from build123d import *

# Parameters (mm, degrees)
F2_R    = 10.6144552681
F3_SIZE = 5


# Not quite as in the source:
# - a feature of the source that left no trace in its solid (it failed there, or was rolled back) is left out


with BuildPart() as f1:
    # F0 (on Front) → F1 (revolve)
    with BuildSketch(Plane.XZ):
        Polygon((-98.2463732362, 0), (0, 0), (0, 76.5963345766), (-31.3552282751, 76.5963345766), (-31.3552282751, 47.6300790906), (-40.9111082554, 47.6300790906), (-40.9111082554, 61.0680393875), (-54.6476840973, 61.0680393875), (-81.5235897899, 42.8521446884), (-81.5235897899, 20.1569329947), (-90.1836082339, 20.1569329947), (-90.1836082339, 39.2686873674), (-98.2463732362, 39.2686873674), align=None)
    revolve(axis=Axis((-49.1231866181, 0, 0), (-1, 0, 0)))

    # F2
    f2_edges = [f1.edges().sort_by_distance(p)[0] for p in [
        (-81.52359, 0, -42.852145),
    ]]
    fillet(f2_edges, radius=F2_R)

    # F3
    f3_edges = [f1.edges().sort_by_distance(p)[0] for p in [
        (-31.355228, 0, -76.596335),
    ]]
    chamfer(f3_edges, length=F3_SIZE)


solid = f1.part
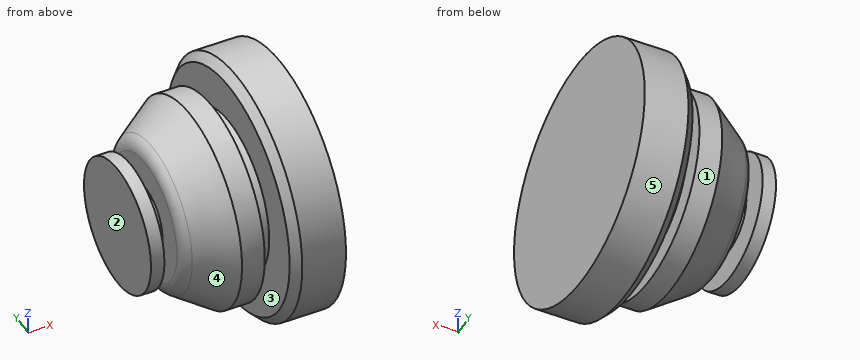
For this review, take the finished solid that the model builds, in its own axes (mm). Face numbers are marked on the shaded views. A direction names the side the tool comes from. Round coordinates to 2 decimals unless told otherwise and drop trailing zeros. Write each loop counter-clockwise with the first axis right and the second up, starting at its lowest first coordinate (ties: lowest second). Pieces come first, ordered by that corner, then holes. Notation, with made-up numbers: (-19, 78) -> (35, 78) arc R17 cw to (35, 95) -> close; hole circle Ø8 at (23, 76.5). An arc over 180 degrees is marked (long way). Use CSV: the item, a comma, the result in double quotes.
(1) Draft analysis for pull direction X (two halves, no side actions). For the marked faces 3, 4 and 5, state which applies: +X half, -X half, draft (parallel to the pull), parting line (faces both ways), or undercut.
Computed values:
face 3,"undercut"
face 4,"-X half"
face 5,"draft"
(2) Clearance check with flat-ended pins moving along their axes: P1, Ø2, axis at y = -41, z = 15.5, coming from the -X side; P2, Ø5, axis at x = -46.5, z = 1.5, coming from the -Y side; P3, Ø10, axis at x = -44, z = -8.5, coming from the +Y side; P4, Ø2, axis at y = -3.5, z = -20, coming from the +X side. State where each tip first meets the part, or that it passes through.
Computed values:
P1,"x = -79.92"
P2,"y = -61.07"
P3,"y = 60.97"
P4,"x = 0"
(3) Consider section A-A, the plane z = 0. Give the boundary of the cut face in (x, y).
Computed values:
outline,"(-98.25, -39.27) -> (-90.18, -39.27) -> (-90.18, -20.16) -> (-81.52, -20.16) -> (-81.52, -37.22) arc R10.61 ccw to (-76.86, -46.01) -> (-54.65, -61.07) -> (-40.91, -61.07) -> (-40.91, -47.63) -> (-31.36, -47.63) -> (-31.36, -71.6) -> (-26.36, -76.6) -> (0, -76.6) -> (0, 76.6) -> (-26.36, 76.6) -> (-31.36, 71.6) -> (-31.36, 47.63) -> (-40.91, 47.63) -> (-40.91, 61.07) -> (-54.65, 61.07) -> (-76.86, 46.01) arc R10.61 ccw to (-81.52, 37.22) -> (-81.52, 20.16) -> (-90.18, 20.16) -> (-90.18, 39.27) -> (-98.25, 39.27) -> close"
(4) For the marked faces 1 and 2, list the 3-axis set-ups (+Z, -Z, +X, -X, +Y, -Y) from which the entire face can be reached by the end or side of a thin tool; tool diameter is ignored.
Computed values:
face 1,"-X"
face 2,"+Z, -Z, -X, +Y, -Y"
(5) To check wall thickness, follow L1, parallel to X at y = -5.5, z = 27; L2, parallel to X at y = 43, z = 27; L3, parallel to Z at x = -41, y = -2. State the ranges of each line that lie inside material, in increasing order. Write a range as [from, to].
Computed values:
L1,"[-98.25, -90.18], [-81.52, 0]"
L2,"[-69.84, -40.91], [-31.36, 0]"
L3,"[-61.04, 61.04]"
(6) Consider section C-C, the plane x = -72.5. Give the boundary of the cut face in (y, z).
Computed values:
outline,"circle Ø97.94 at (0, 0)"
